from build123d import *

# Parameters (mm, degrees)
BOSS_EXTRUDE1_DEPTH = 3


with BuildPart() as part:
    # Sketch1 → Boss-Extrude1 (new body)
    with BuildSketch(Plane(origin=(0, 0, 0), x_dir=(0, 0, -1), z_dir=(1, 0, 0))):
        Polygon((7.4, 0), (-7.4, 0), (-7.4, -3), (-47.6, -3), (-47.6, 0), (-62.4, 0), (-62.4, -3), (-102.6, -3), (-102.6, 0), (-117.4, 0), (-117.4, -3), (-157.6, -3), (-157.6, 0), (-172.4, 0), (-172.4, -3), (-189.7, -3), (-189.7, -12.8), (-186.7, -12.8), (-186.7, -23.1), (-189.7, -23.1), (-189.7, -28), (-189.7, -32.9), (-186.7, -32.9), (-186.7, -43.2), (-189.7, -43.2), (-189.7, -53), (-172.4, -53), (-172.4, -56), (-157.6, -56), (-157.6, -53), (-117.4, -53), (-117.4, -56), (-102.6, -56), (-102.6, -53), (-62.4, -53), (-62.4, -56), (-47.6, -56), (-47.6, -53), (-7.4, -53), (-7.4, -56), (7.4, -56), (7.4, -53), (47.6, -53), (47.6, -56), (62.4, -56), (62.4, -53), (102.6, -53), (102.6, -56), (117.4, -56), (117.4, -53), (157.6, -53), (157.6, -56), (172.4, -56), (172.4, -53), (189.7, -53), (189.7, -43.2), (186.7, -43.2), (186.7, -32.9), (189.7, -32.9), (189.7, -28), (189.7, -23.1), (186.7, -23.1), (186.7, -12.8), (189.7, -12.8), (189.7, -3), (172.4, -3), (172.4, 0), (157.6, 0), (157.6, -3), (117.4, -3), (117.4, 0), (102.6, 0), (102.6, -3), (62.4, -3), (62.4, 0), (47.6, 0), (47.6, -3), (7.4, -3), align=None)
    extrude(amount=BOSS_EXTRUDE1_DEPTH)


solid = part.part
Design review of the part built by this model. Coordinates are the model's own, in mm. Round coordinates to 2 decimals unless told otherwise and drop trailing zeros. Order: outer loops, then holes, each group sorted by start corner. A loop starts at its lowest first (then second) coordinate and runs counter-clockwise, first axis right, second up. Notation, with made-up numbers: M 85.5,53 L 122.5,53 A29 cw 122.5,78 Z; hole C -40,28 d4. An arc over 180 degrees is marked long. Answer as CSV lines item,"result". Start each with the question number.
1) For pin 1 Ø0.9 at (x, y) = (1.5, -2) entering from +Z; pin 2 Ø0.9 at (x, y) = (1.5, -2) entering from -Z; pin 3 Ø0.9 at (x, z) = (1.5, 76) entering from -Y, all flat-tipped, find the tip position at first contact; note any pin that passes through.
2) Wall thickness on line 1 along Y through (x, z) = (1.55, 85.5); line 2 along Z through (x, y) = (1, -39.5): over which ranges is each line inside the solid? List them lowest first. Write a range as [from, to].
3) Add section A-A (z = 84). Give the boundary of the cut face in (x, y), then the cut area to 3 significant figures.
Resolved:
1,pin 1,"z = 172.4"
1,pin 2,"z = -172.4"
1,pin 3,"y = -53"
2,line 1,"[-53, -3]"
2,line 2,"[-186.7, 186.7]"
3,outline,"M 0,-53 L 3,-53 L 3,-3 L 0,-3 Z"
3,area,"150 mm^2"
